Input: part model. Units: mm. Frame: model coordinates. A direction names the side the tool comes from. Coordinates: 2 decimals unless noted, no trailing zeros. Write each loop counter-clockwise with the first axis right and the second up, starting at its lowest first coordinate (ties: lowest second). Pieces come first, ordered by that corner, then holes. Notation, with made-up numbers: (30.25, -5) - (52.25, -5) arc R29 cw to (52.25, 15) - close; hole circle Ø2 at (40, -32.5). An arc over 180 degrees is marked (long way). Use CSV: the item, a comma, the result in double quotes.
```python
from build123d import *

# Parameters (mm, degrees)
F1_DEPTH   = 6.35
F2_DEPTH   = 25.4
F3_DEPTH   = 50.8
F4_SIZE2   = 10.9985226281
F4_SIZE    = 6.35
F4_2_SIZE2 = 10.9985226281
F4_2_SIZE  = 6.35
F5_SIZE2   = 7.3323484187
F5_SIZE    = 12.7
F6_R       = 6.34999


# Not quite as in the source:
# - a fillet or chamfer is up to 0.001 mm smaller than in the source, because OpenCascade refuses the exact size


with BuildPart() as f1:
    # F0 (on Top) → F1 (new body)
    with BuildSketch(Plane.XY):
        Polygon((-50.1812659204, 67.9668266764), (-50.1812659204, -97.5199052306), (38.7187340796, -97.1034997316), (38.7187340796, 67.9668266764), align=None)
        Polygon((-5.7312659204, -90.7831733236), (-43.8312659204, -90.7831733236), (-43.8312659204, 23.5168266764), (-43.8312659204, 61.6168266764), (-5.7312659204, 61.6168266764), (32.3687340796, 61.6168266764), (32.3687340796, -52.6831733236), (32.3687340796, -90.7831733236), align=None, mode=Mode.SUBTRACT)
    extrude(amount=F1_DEPTH)

    # F0 (on Top) → F2 (join)
    with BuildSketch(Plane.XY):
        with BuildLine():
            Line((-43.8312659204, 23.5168266764), (-43.8312659204, -90.7831733236))
            Line((-43.8312659204, -90.7831733236), (-5.7312659204, -90.7831733236))
            Line((-5.7312659204, -90.7831733236), (-5.7312659204, -65.3831733236))
            ThreePointArc((-5.7312659204, -65.3831733236), (-2.0115220415, -56.4029172025), (6.9687340796, -52.6831733236))
            Line((6.9687340796, -52.6831733236), (32.3687340796, -52.6831733236))
            Line((32.3687340796, -52.6831733236), (32.3687340796, 61.6168266764))
            Line((32.3687340796, 61.6168266764), (-5.7312659204, 61.6168266764))
            Line((-5.7312659204, 61.6168266764), (-5.7312659204, 36.2168266764))
            ThreePointArc((-5.7312659204, 36.2168266764), (-9.4510097993, 27.2365705553), (-18.4312659204, 23.5168266764))
            Line((-18.4312659204, 23.5168266764), (-43.8312659204, 23.5168266764))
        make_face()
    extrude(amount=F2_DEPTH)

    # F0 (on Top) → F3 (join)
    with BuildSketch(Plane.XY):
        with BuildLine():
            Line((-43.8312659204, 61.6168266764), (-43.8312659204, 23.5168266764))
            Line((-43.8312659204, 23.5168266764), (-18.4312659204, 23.5168266764))
            ThreePointArc((-18.4312659204, 23.5168266764), (-9.4510097993, 27.2365705553), (-5.7312659204, 36.2168266764))
            Line((-5.7312659204, 36.2168266764), (-5.7312659204, 61.6168266764))
            Line((-5.7312659204, 61.6168266764), (-43.8312659204, 61.6168266764))
        make_face()
        with BuildLine():
            Line((-5.7312659204, -65.3831733236), (-5.7312659204, -90.7831733236))
            Line((-5.7312659204, -90.7831733236), (32.3687340796, -90.7831733236))
            Line((32.3687340796, -90.7831733236), (32.3687340796, -52.6831733236))
            Line((32.3687340796, -52.6831733236), (6.9687340796, -52.6831733236))
            ThreePointArc((6.9687340796, -52.6831733236), (-2.0115220415, -56.4029172025), (-5.7312659204, -65.3831733236))
        make_face()
    extrude(amount=F3_DEPTH)

    # F4
    f4_edges = [f1.edges().sort_by_distance(p)[0] for p in [
        (13.318734, -90.783173, 50.8),
    ]]
    f4_side = f1.faces().sort_by_distance((13.714776, -72.129216, 50.8))[0]
    chamfer(f4_edges, length=F4_SIZE, length2=F4_SIZE2, reference=f4_side)

    # F4#2
    f4_2_edges = [f1.edges().sort_by_distance(p)[0] for p in [
        (-43.831266, 42.566827, 50.8),
    ]]
    f4_2_side = f1.faces().sort_by_distance((-43.831266, -0.295673, 21.43125))[0]
    chamfer(f4_2_edges, length=F4_2_SIZE, length2=F4_2_SIZE2, reference=f4_2_side)

    # F5
    f5_edges = [f1.edges().sort_by_distance(p)[0] for p in [
        (32.368734, 4.466827, 25.4),
        (-24.781266, -90.783173, 25.4),
        (-43.831266, -33.633173, 25.4),
        (13.318734, 61.616827, 25.4),
    ]]
    f5_side = f1.faces().sort_by_distance((-5.731266, -14.583173, 25.4))[0]
    chamfer(f5_edges, length=F5_SIZE, length2=F5_SIZE2, reference=f5_side)

    # F6 (radius 6.35 in the source; OpenCascade refuses exactly that, so slightly less here)
    f6_edges = [f1.edges().sort_by_distance(p)[0] for p in [
        (38.718734, -14.568337, 6.35),
        (-5.731266, -97.311702, 6.35),
        (-5.731266, 67.966827, 6.35),
        (-50.181266, -14.776539, 6.35),
    ]]
    fillet(f6_edges, radius=F6_R)


solid = f1.part
```
(1) Cut plane C-C on z = 14. Return loops of the section in (x, y), and give its area (3 significant figures).
Check values:
outline,"(-43.83, -90.78) - (32.37, -90.78) - (32.37, 61.62) - (-43.83, 61.62) - close"
area,"11,600 mm^2"
(2) Pin query (flat end, axial travel): pin 1 Ø1 at (x, z) = (-7, 5.5) entering from +Y; pin 2 Ø1.5 at (x, z) = (-11, 37.5) entering from -Y; pin 3 Ø5 at (y, z) = (-48.5, 35.5) entering from +X; pin 4 Ø2 at (y, z) = (25, 20.5) entering from +X. Return the tip coordinate at first contact, or that it passes through.
Check values:
pin 1,"y = 65.53"
pin 2,"y = 25.42"
pin 3,"through"
pin 4,"x = 29.89"
(3) Ray query, probe 1 along Z at (x, y) = (2, -9); probe 2 along Y at (x, z) = (-43, 37); probe 3 along X at (y, z) = (-70, 7.5). Return the intervals inside material, ascending. Write a range as from..to.
Check values:
probe 1,"0..25.4"
probe 2,"23.52..61.62"
probe 3,"-43.83..32.37"
(4) Reachability of faces 1 (the cylindrical face through (-5.12, -95.4, 4.54)), 2 (the flat face through (-14, 61.617, 23)), 3 (the flat face through (-37.57, -32.833, 21.682)) from +Z, -Z, +X, -X, +Y, -Y: full face, straight path, thin tool, end or side. Return the list, or none.
Check values:
face 1,"+Z, +X, -Y"
face 2,"+Z, +X, -X, +Y"
face 3,"+Z, -X, -Y"
(5) Cut plane A-A on z = 37.5. Return loops of the section in (x, y), and give its area (3 significant figures).
Check values:
outline,"(-43.83, 23.52) - (-18.43, 23.52) arc R12.7 ccw to (-5.73, 36.22) - (-5.73, 61.62) - (-43.83, 61.62) - close; (-5.73, -90.78) - (32.37, -90.78) - (32.37, -52.68) - (6.97, -52.68) arc R12.7 ccw to (-5.73, -65.38) - close"
area,"2,830 mm^2"
